Print and shaded views of the part. All mm, measured from the part's lowest x, y and z. Give positions to 0.01 mm unless a question says otherwise; leave off trailing zeros. Loops run counter-clockwise (first coordinate to the right, second up) from the corner with the lowest first, then second, coordinate; pieces in that order, holes last.
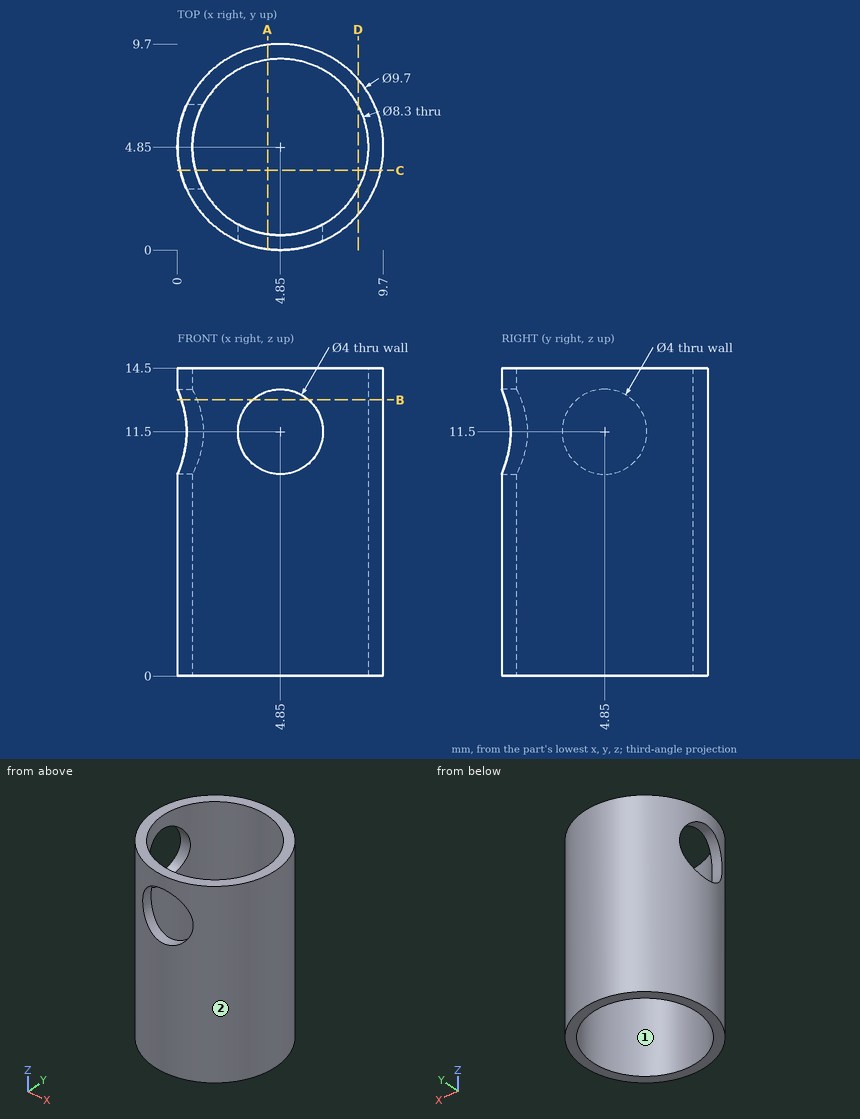
1. Pull direction Y, two halves, no side cores. Call the marked faces 1 and 2: released by +Y, released by -Y, zero draft, split by the parting line, or undercut.
Responses:
face 1: undercut
face 2: split by the parting line
2. Saw through at D-D, the plane x = 8.5. List the corners of the cut face in (y, z), and give its area (3 significant figures).
Responses:
outline: (1.66, 0) - (2.88, 0) - (2.88, 14.5) - (1.66, 14.5) - close; (6.82, 0) - (8.04, 0) - (8.04, 14.5) - (6.82, 14.5) - close
area: 35.3 mm2
3. Drop flat-ended pins along their axis: pin 1 (3 mm diameter, centred on y = 7.5, z = 5, fed in from -X); pin 2 (4.5 mm diameter, centred on y = 4.85, z = 11.5, fed in from -X). Give the stop position or say it passes through.
Responses:
pin 1: stops at x = 0.14
pin 2: stops at x = 0
4. Saw through at B-B, the plane z = 13. List the corners of the cut face in (x, y), and give its area (3 significant figures).
Responses:
outline: (0.18, 3.53) arc R4.85 ccw to (3.53, 0.18) - (3.53, 0.92) arc R4.15 cw to (0.92, 3.53) - close; (0.18, 6.17) - (0.92, 6.17) arc R4.15 cw (long way) to (6.17, 0.92) - (6.17, 0.18) arc R4.85 ccw (long way) to start
area: 16.0 mm2
5. Saw through at C-C, the plane y = 3.75. List the corners of the cut face in (x, z), and give its area (3 significant figures).
Responses:
outline: (0.13, 0) - (0.85, 0) - (0.85, 9.83) - (0.13, 9.83) - close; (0.13, 13.17) - (0.85, 13.17) - (0.85, 14.5) - (0.13, 14.5) - close; (8.85, 0) - (9.57, 0) - (9.57, 14.5) - (8.85, 14.5) - close
area: 18.5 mm2
6. Saw through at A-A, the plane x = 4.25. List the corners of the cut face in (y, z), and give its area (3 significant figures).
Responses:
outline: (0.04, 0) - (0.74, 0) - (0.74, 9.59) - (0.04, 9.59) - close; (0.04, 13.41) - (0.74, 13.41) - (0.74, 14.5) - (0.04, 14.5) - close; (8.96, 0) - (9.66, 0) - (9.66, 14.5) - (8.96, 14.5) - close
area: 17.8 mm2
7. Probe line 1 along Y through (x, z) = (4.75, 9); line 2 along X through (y, z) = (7.75, 6.5); line 3 along Y through (x, z) = (8.5, 12.25). List the from-to ranges inside material, lowest first.
Responses:
line 1: y = 0 to 0.7, 9 to 9.7
line 2: x = 0.96 to 1.88, 7.82 to 8.74
line 3: y = 1.66 to 2.88, 6.82 to 8.04
